Input: dimensioned drawing with shaded views. Units: mm. Origin: part minimum x, y, z. A direction names the side the tool comes from. Give positions to 0.01 mm unless a question says otherwise; leave off trailing zeros. Write each loop counter-clockwise with the first axis right and the second up, starting at its lowest first coordinate (ties: lowest second). Pieces come first, ordered by that corner, then holes. Notation, with made-up numbers: (66.5, 42) -> (77.5, 42) arc R21 cw to (77.5, 46) -> close; hole circle Ø5 at (15.25, 34). An arc over 180 degrees is marked (long way). Return JSON: item names as keys, results as strings. Group by question number.
Item 1: Section A-A, the plane z = 3. Count the separate pieces of the cut face and the enclosed holes in it, then the cut area to 3 significant figures.
Item 2: Pin query (flat end, axial travel): P1, Ø5, axis at x = 13.5, y = 22.5, coming from the -Z side; P2, Ø1.5, axis at x = 19, z = 2, coming from the -Y side; P3, Ø1.5, axis at x = 19.5, z = 2, coming from the +Y side; P4, Ø1.8, axis at y = 12, z = 4, coming from the +X side. Return the tip coordinate at first contact, or that it passes through.
Item 3: Set-up query: the marked faces 4, 5, 6, 7 and 8. Return all of +Z, -Z, +X, -X, +Y, -Y with unobstructed straight access to the full face (end or side cutting, diameter ignored); none if empty.
Item 4: Section C-C, the plane x = 17.5. Return loops of the section in (y, z) (1 decimal).
Item 5: Section D-D, the plane y = 21.5. Return loops of the section in (x, z) (1 decimal).
Item 6: Mould query, pull axis Y, two halves, no side actions, for the marked faces 1, 2 and 3. Classes: released by +Y, released by -Y, zero draft, split by the parting line, or undercut.
Item 7: Line query: line 1 (Z direction, x = 3.8, y = 12.5); line 2 (Y direction, x = 11.25, z = 2.5) (1 decimal); line 3 (X direction, y = 2.25, z = 2.75) (1 decimal). Output: solid intervals per line, ascending. Write a range as [from, to].
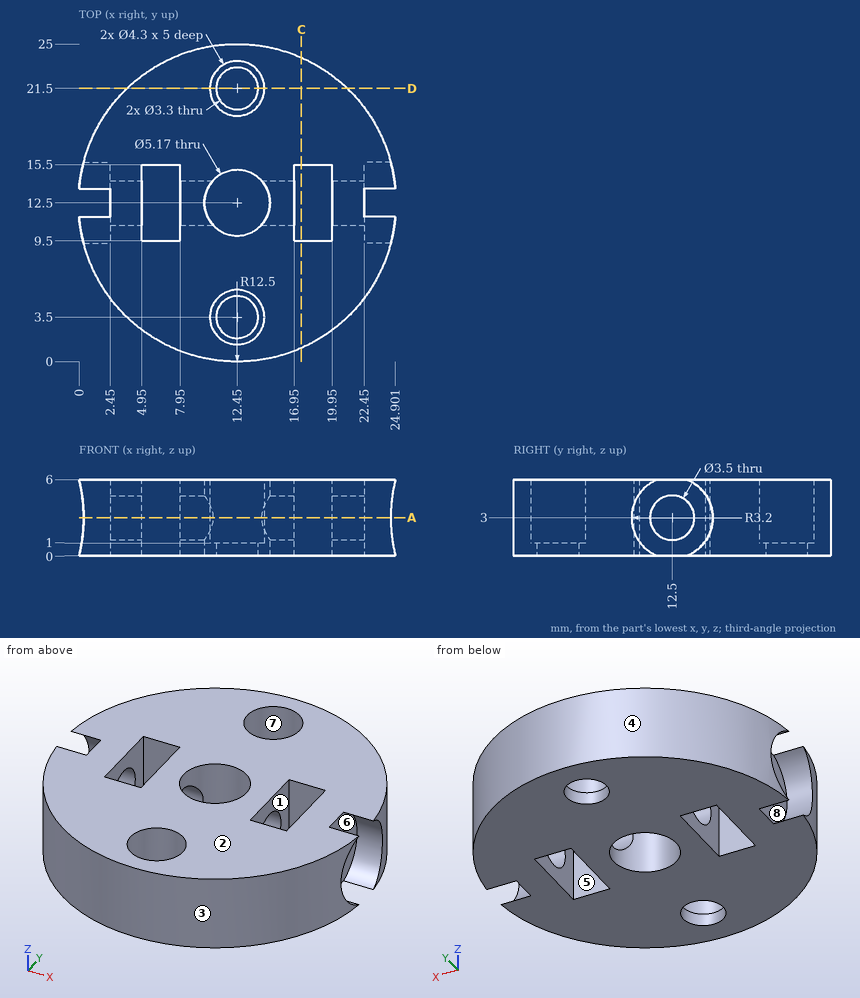
Answer below:
{
 "1": {"separate pieces": "2", "enclosed holes": "2", "area": "342 mm2"},
 "2": {"P1": "stops at z = 0", "P2": "stops at y = 1.43", "P3": "stops at y = 23.3", "P4": "stops at x = 22.45"},
 "3": {"face 4": "+Z, -Z, +Y", "face 5": "+Z, -Z", "face 6": "+X", "face 7": "+Z", "face 8": "-X"},
 "4": {"outline": "(1.1, 0) -> (9.5, 0) -> (9.5, 6) -> (1.1, 6) -> close; (15.5, 0) -> (23.9, 0) -> (23.9, 6) -> (15.5, 6) -> close"},
 "5": {"outline": "(3.8, 0) -> (10.8, 0) -> (10.8, 1) -> (10.3, 1) -> (10.3, 6) -> (3.8, 6) -> close; (14.1, 0) -> (21.1, 0) -> (21.1, 6) -> (14.6, 6) -> (14.6, 1) -> (14.1, 1) -> close"},
 "6": {"face 1": "undercut", "face 2": "zero draft", "face 3": "released by -Y"},
 "7": {"line 1": "z = [0, 1.25], [4.75, 6]", "line 2": "y = [0.1, 1.7], [5.3, 10.2], [14.8, 19.7], [23.3, 24.9]", "line 3": "x = [5.3, 10.7], [14.2, 19.6]"}
}
